```python
from build123d import *

# Parameters (mm, degrees)
SHELL4_T           = -1
FILLET3_R          = 1
CHAMFER1_SIZE      = 0.5
SKETCH14_RX        = 2.2
SKETCH14_RY        = 1.7
CUT_EXTRUDE1_DEPTH = 8


with BuildPart() as part:
    # Sketch9 → Revolve4 (revolve)
    with BuildSketch(Plane.XY, mode=Mode.PRIVATE) as revolve4_sk:
        with BuildLine():
            Line((0, 0), (12.5, 0))
            ThreePointArc((12.5, 0), (9.435034301, 4.435034301), (5, 7.5))
            Line((5, 7.5), (0, 7.5))
            Line((0, 7.5), (0, 0))
        make_face()
    revolve(revolve4_sk.sketch.rotate(Axis((0, 0, 0), (0, 1, 0)), 90), axis=Axis((0, 0, 0), (0, 1, 0)))

    # Shell4
    shell4_openings = [part.faces().sort_by_distance(p)[0] for p in [
        (0, 0, 0),
    ]]
    offset(amount=SHELL4_T, openings=shell4_openings, kind=Kind.INTERSECTION)

    # Sketch10 → Revolve5 (revolve)
    with BuildSketch(Plane.XY, mode=Mode.PRIVATE) as revolve5_sk:
        Polygon((0, 47.5), (0, 7.5), (2.75, 7.5), (5, 7.5), (7.5, 47.5), align=None)
        Polygon((2.75, 7.5), (0, 7.5), (0, 1.5), (2.75, 1.5), (2.75, 4.5), align=None)
    revolve(revolve5_sk.sketch.rotate(Axis((0, 7.5, 0), (0, 1, 0)), 90), axis=Axis((0, 7.5, 0), (0, 1, 0)))

    # Fillet3
    fillet3_edges = [part.edges().sort_by_distance(p)[0] for p in [
        (0, 47.5, 7.5),
    ]]
    fillet(fillet3_edges, radius=FILLET3_R)

    # Chamfer1
    # the kernel refuses this chamfer: 0.859778685, 0.5 mm, written as the material it adds along each edge
    with BuildSketch(Plane(origin=(0, 7.5, 0), x_dir=(0, 0, -1), z_dir=(1, 0, 0))) as chamfer1_piece_1:
        with BuildLine():
            Line((5 + CHAMFER1_SIZE * 0.0623782861552, CHAMFER1_SIZE * 0.998052578483), (5.829343974, -0.405549185))
            ThreePointArc((5.829343974, -0.405549185), (5.432071901, -0.203384623), (5, 0))
            Line((5, 0), (5 + CHAMFER1_SIZE * 0.0623782861552, CHAMFER1_SIZE * 0.998052578483))
        make_face()
    revolve(axis=Axis((0, 7.5, 0), (0, 1, 0)))

    # Sketch13 → Revolve6 (revolve)
    with BuildSketch(Plane.XY, mode=Mode.PRIVATE) as revolve6_sk:
        Polygon((5, 7.5), (2.75, 4.5), (2.75, 7.5), align=None)
    revolve(revolve6_sk.sketch.rotate(Axis((0, 7.5, 0), (0, -1, 0)), 270), axis=Axis((0, 7.5, 0), (0, -1, 0)))

    # Sketch14 → Cut-Extrude1 (cut)
    with BuildSketch(Plane.XZ.offset(-1.5)):
        with Locations((0, 0)):
            Ellipse(SKETCH14_RX, SKETCH14_RY)
    extrude(amount=-CUT_EXTRUDE1_DEPTH, mode=Mode.SUBTRACT)


solid = part.part
```
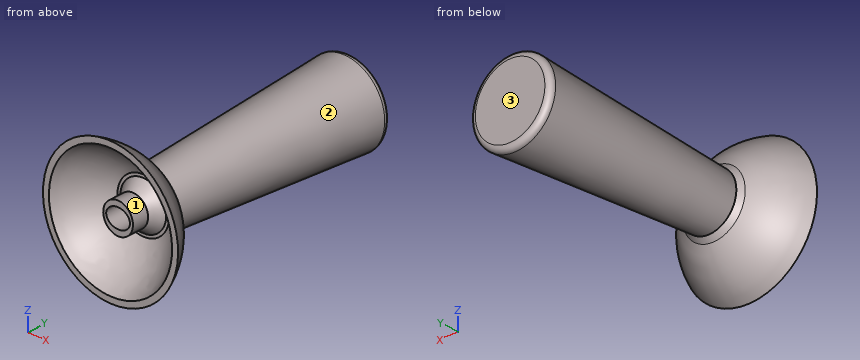
CAD build for the part. Positions are in the model's coordinates, mm. Face numbers are marked on the shaded views. Round coordinates to 2 decimals unless told otherwise and drop trailing zeros. Order: outer loops, then holes, each group sorted by start corner. A loop starts at its lowest first (then second) coordinate and runs counter-clockwise, first axis right, second up. Notation, with made-up numbers: (64, 7.25) -> (73, 7.25) arc R30 ccw to (73, 30.25) -> close; hole circle Ø1 at (-8, -35). An arc over 180 degrees is marked (long way). One line per question, with ' | ' between items.
Q1. Slice it at A-A (y = 6). Give the number of separate pieces and of enclosed holes in the cut face, then the cut area to 3 significant figures.
Completed:
separate pieces: 2 | enclosed holes: 2 | area: 113 mm^2
Q2. Drop flat-ended pins along their axis: pin 1 (12 mm diameter, centred on x = -8, z = 6.5, fed in from +Y); pin 2 (3 mm diameter, centred on x = 3.5, z = -9, fed in from +Y); pin 3 (6 mm diameter, centred on y = 23, z = 1.5, fed in from -X); pin 4 (10.5 mm diameter, centred on x = 1.5, z = 1, fed in from -Y). Give the stop position or say it passes through.
Completed:
pin 1: stops at y = 47.5 | pin 2: stops at y = 5.58 | pin 3: stops at x = -6.13 | pin 4: stops at y = 1.5
Q3. Two-plate mould, pull along Z, no slides. Class the marked faces 1, 2 and 3: released by +Z, released by -Z, zero draft, split by the parting line, or undercut.
Completed:
face 1: undercut | face 2: split by the parting line | face 3: zero draft
Q4. Slice it at B-B (y = 11). Write the cut outline in (x, z).
Completed:
outline: circle Ø10.44 at (0, 0)
Q5. Slice it at C-C (y = 39). Write the cut outline in (x, z), then the cut area to 3 significant figures.
Completed:
outline: circle Ø13.94 at (0, 0) | area: 153 mm^2
Q6. Probe probe 1 along Z at (x, y) = (2.5, 6); probe 2 along X at (y, z) = (5, 0.5); probe 3 along Z at (x, y) = (-1.75, 4). List the from-to ranges inside material, lowest first.
Completed:
probe 1: z = -7.17 to -5.17, -2.96 to 2.96, 5.17 to 7.17 | probe 2: x = -8.82 to -7.25, -3.08 to -2.1, 2.1 to 3.08, 7.25 to 8.82 | probe 3: z = -9.7 to -8.26, -2.12 to -1.03, 1.03 to 2.12, 8.26 to 9.7
